The listing builds one solid part. Answer for the finished solid, in the listing's coordinates (mm). Face numbers are marked on the shaded views. A direction names the side the tool comes from. Give positions to 0.01 mm unless a question says otherwise; leave off trailing zeros. Order: outer loops, then holes, each group sorted by start corner. A loop starts at its lowest first (then second) coordinate and runs counter-clockwise, first axis right, second up. Notation, with made-up numbers: (37.25, 19.25) - (95.25, 19.25) arc R15 ccw to (95.25, 24.25) - close; hole circle Ø6 at (-34.75, -7.5). An arc over 180 degrees is marked (long way). Use a Markdown table: item, result. Add a question column.
1) Flat-ended cylindrical pins translate along their axes: pin 1 (1.5 mm diameter, centred on x = -2, z = 12.5, fed in from +Y); pin 2 (4 mm diameter, centred on y = 3, z = 16.5, fed in from +X); pin 3 (5 mm diameter, centred on x = -6, z = 10.5, fed in from -Y). Find the tip coordinate at first contact, or state that the pin passes through.
2) Find section A-A, the plane z = 20.75. Determine the outline of the cut face in (x, y), plus the area to 3 significant figures.
3) Find section C-C, the plane y = 5.5. Determine the outline of the cut face in (x, z), plus the area to 3 significant figures.
4) Straight lines are drawn through the part: line 1 (X direction, y = 4.25, z = 4.5); line 2 (X direction, y = -8.5, z = 20); line 3 (Y direction, x = -6.5, z = 3). For each, find the intervals that lie inside material, in ascending order.
5) Find section B-B, the plane x = -6. Determine the outline of the cut face in (y, z).
6) For the marked faces 1 and 2, determine the directions among +Z, -Z, +X, -X, +Y, -Y from which every point of the face is accessible in a straight line to the end or side of a thin tool.
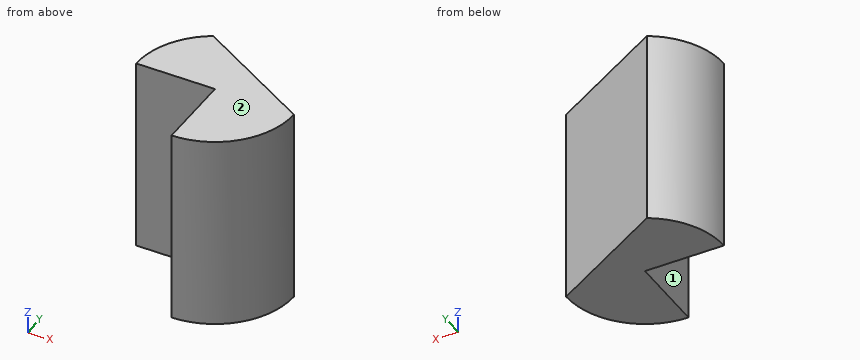
from build123d import *

# Parameters (mm, degrees)
BOSS_EXTRUDE1_DEPTH = 25


with BuildPart() as part:
    # Sketch1 → Boss-Extrude1 (new body)
    with BuildSketch(Plane.XY):
        with BuildLine():
            Line((-10, 0), (0, 0))
            Line((0, 0), (0, -10))
            ThreePointArc((0, -10), (7.071067812, -7.071067812), (10, 0))
            Line((10, 0), (-5, 8.660254038))
            ThreePointArc((-5, 8.660254038), (-8.660254038, 5), (-10, 0))
        make_face()
    extrude(amount=BOSS_EXTRUDE1_DEPTH)


solid = part.part
The answers:
| question | item | result |
|---|---|---|
| 1 | pin 1 | y = 7.36 |
| 1 | pin 2 | x = 8.27 |
| 1 | pin 3 | y = 0 |
| 2 | outline | (-10, 0) - (0, 0) - (0, -10) arc R10 ccw to (10, 0) - (-5, 8.66) arc R10 ccw to start |
| 2 | area | 174 mm2 |
| 3 | outline | (-8.35, 0) - (0.47, 0) - (0.47, 25) - (-8.35, 25) - close |
| 3 | area | 221 mm2 |
| 4 | line 1 | -9.05 to 2.64 |
| 4 | line 2 | 0 to 5.27 |
| 4 | line 3 | 0 to 7.6 |
| 5 | outline | (0, 0) - (8, 0) - (8, 25) - (0, 25) - close |
| 6 | face 1 | +Z, -Z, -X, -Y |
| 6 | face 2 | +Z, +X, -X, +Y, -Y |
